Autodesk Fusion 360 part; units mm, degrees
sketch "Sketch7" plane through (0, 0, 0) normal (0, 1, 0) x (1, 0, 0)
  line L0 (2455.4576, -95.8693) -> (2455.4576, -76.2)
  line L1 (2455.4576, -76.2) -> (2651.76, 0)
  line L2 (2651.76, 0) -> (2706.624, 0)
  line L3 (2706.624, 0) -> (3456.432, -140.208)
  line L4 (3456.432, -140.208) -> (3535.68, -408.432)
  line L5 (3535.68, -408.432) -> (3066.288, -402.336)
  line L6 (3066.288, -402.336) -> (2455.4576, -95.8693)
extrude "Extrude5" add sketch "Sketch7" along normal blind 950.976
sketch "Sketch8" plane through (0, 0, 0) normal (1, 0, 0) x (0, 1, 0)
  line L0 (950.976, 426.72) -> (0, 426.72)
  line L1 (475.488, 426.72) -> (475.488, -243.84)
  line L2 (1005.84, 457.2) -> (-54.0718, 457.2)
  line L3 (-54.0718, 457.2) -> (-54.0718, -231.5284)
  line L4 (-54.0718, -231.5284) -> (1005.84, -231.5284)
  line L5 (1005.84, -231.5284) -> (1005.84, 457.2)
  line L6 (911.352, 27.432) -> (933.2048, 2.8476)
  line L7 (938.5836, 2.5312) -> (943.1535, 6.5933)
  line L8 (944.4292, 9.2894) -> (950.976, 173.736)
  line L9 (950.976, 173.736) -> (950.976, 391.668)
  line L10 (917.448, 391.668) -> (902.208, 176.784)
  line L11 (902.208, 176.784) -> (475.488, 176.784)
  arc A0 (950.976, 391.668) -> (917.448, 391.668) centre (934.212, 391.668) ccw
  line L12 (911.352, 27.432) -> (475.488, 27.432)
  arc A1 (933.2048, 2.8476) -> (938.5836, 2.5312) centre (936.0524, 5.3789) ccw
  arc A2 (943.1535, 6.5933) -> (944.4292, 9.2894) centre (940.6223, 9.4409) ccw
  line L13 (48.768, 176.784) -> (475.488, 176.784)
  line L14 (33.528, 391.668) -> (48.768, 176.784)
  arc A3 (33.528, 391.668) -> (0, 391.668) centre (16.764, 391.668) ccw
  line L15 (0, 173.736) -> (0, 391.668)
  line L16 (6.5468, 9.2894) -> (0, 173.736)
  arc A4 (6.5468, 9.2894) -> (7.8225, 6.5933) centre (10.3537, 9.4409) ccw
  line L17 (12.3924, 2.5312) -> (7.8225, 6.5933)
  arc A5 (12.3924, 2.5312) -> (17.7712, 2.8476) centre (14.9236, 5.3789) ccw
  line L18 (39.624, 27.432) -> (17.7712, 2.8476)
  line L19 (39.624, 27.432) -> (475.488, 27.432)
  dimension "d19" = 3.81
extrude "Extrude6" cut sketch "Sketch8" along normal blind 3962.4
ref_plane "WorkPlane3" through (3041.9851, 475.488, 481.584) normal (0, 0, 1) x (0, -1, 0)
sketch "Sketch10" plane through (0, 0, 481.584) normal (0, 0, 1) x (-1, 0, 0)
  line L0 (-2616.7317, -902.208) -> (-2616.7317, -48.768)
  line L1 (-2616.7317, -48.768) -> (-3467.2386, -48.768)
  line L2 (-3467.2386, -48.768) -> (-3467.2386, -902.208)
  line L3 (-3467.2386, -902.208) -> (-2616.7317, -902.208)
  line L4 (-2616.7317, -475.488) -> (-3627.1201, -475.488)
  line L5 (-2616.7317, -475.488) -> (-2616.7317, -932.688)
  line L6 (-2616.7317, -932.688) -> (-3467.2386, -902.208)
  line L7 (-3467.2386, -902.208) -> (-3467.2386, -475.488)
  line L8 (-2616.7317, -475.488) -> (-2616.7317, -18.288)
  line L9 (-2616.7317, -18.288) -> (-3467.2386, -48.768)
  line L10 (-3467.2386, -48.768) -> (-3467.2386, -475.488)
extrude "Extrude7" cut sketch "Sketch10" against normal blind 304.8 contours L3 L5 L6 | L1 L8 L9
Geometry: final body of the model. Coordinates: model frame, mm. A direction names the side the tool comes from. Give positions to 0.01 mm unless a question says otherwise; leave off trailing zeros. Loops run counter-clockwise (first coordinate to the right, second up) from the corner with the lowest first, then second, coordinate; pieces in that order, holes last. Notation, with made-up numbers: (-18, -3.75) -> (23, -3.75) arc R18 ccw to (23, 27.25) -> close; hole circle Ø11 at (48.25, 54.5). An arc over 180 degrees is marked (long way). Use CSV: the item, a comma, the result in double quotes.
(1) First-contact query: P1, Ø2, axis at y = 307.5, z = 103.5, coming from the -X side; P2, Ø8, axis at y = 648, z = 151.5, coming from the +X side; P3, Ø1.5, axis at x = 2607.5, z = 58, coming from the +Y side. Flat tips, straight axial feed; report the tip coordinate or a pass-through.
From the geometry:
P1,"x = 2468.67"
P2,"x = 3460.95"
P3,"y = 946.4"
(2) Ray query, line 1 along Z through (x, y) = (2748, 650.5); line 2 along Z through (x, y) = (2969, 797); line 3 along Y through (x, z) = (3460, 222.5). Return the intervals inside material, ascending. Write a range as [from, to].
From the geometry:
line 1,"[27.43, 176.78]"
line 2,"[49.06, 176.78]"
line 3,"[0, 45.53], [905.45, 950.98]"
(3) Cut plane C-C (y = 872). Output: boundary loops of the cut face in (x, z), plus the area to 3 significant figures.
From the geometry:
outline,"(2455.46, 76.2) -> (2581.09, 27.43) -> (2853.33, 27.43) -> (3456.43, 140.21) -> (3467.24, 176.78) -> (2616.73, 176.78) -> (2455.46, 95.87) -> close"
area,"106,000 mm^2"
(4) Cut plane D-D (z = 271). Output: boundary loops of the cut face in (x, y), plus the area to 3 significant figures.
From the geometry:
outline,"(2804.52, 0) -> (3495.08, 0) -> (3495.08, 42.09) -> (3280.79, 42.09) -> (2804.52, 25.02) -> close; (2804.52, 925.96) -> (3280.79, 908.89) -> (3495.08, 908.89) -> (3495.08, 950.98) -> (2804.52, 950.98) -> close"
area,"50,000 mm^2"
(5) Cut plane A-A (z = 197). Output: boundary loops of the cut face in (x, y).
From the geometry:
outline,"(2657.03, 0) -> (3473.21, 0) -> (3473.21, 47.33) -> (3427.23, 47.33) -> (2657.03, 19.73) -> close; (2657.03, 931.24) -> (3427.23, 903.64) -> (3473.21, 903.64) -> (3473.21, 950.98) -> (2657.03, 950.98) -> close"
(6) Cut plane B-B (x = 3328). Output: boundary loops of the cut face in (y, z).
From the geometry:
outline,"(0, 173.74) -> (2.29, 116.19) -> (948.69, 116.19) -> (950.98, 173.74) -> (950.98, 391.67) arc R16.76 ccw to (943.33, 405.73) -> (925.09, 405.73) arc R16.76 ccw to (917.45, 391.67) -> (907.2, 247.14) -> (907.2, 176.78) -> (43.78, 176.78) -> (43.78, 247.14) -> (33.53, 391.67) arc R16.76 ccw to (25.88, 405.73) -> (7.65, 405.73) arc R16.76 ccw to (0, 391.67) -> close"
(7) Pull-direction query (Y, two-part tool) for faces 1 (the face through (2841.502, 948.384, 108.633)), 2 (the face through (3048, 469, 176.784)), 3 (the face through (2528.88, 468.89, 47.7)); classes: released by +Y, released by -Y, zero draft, split by the parting line, or undercut.
From the geometry:
face 1,"released by +Y"
face 2,"undercut"
face 3,"zero draft"
(8) Access query for faces 4 (the face through (3337.84, 913.32, 333.48)), 5 (the face through (2715.303, 31.279, 18.043)), 6 (the face through (2841.5, 2.59, 108.63)). Directions: +Z, -Z, +X, -X, +Y, -Y. A direction counts if a zero-diameter tool reaches every point of the face in a straight line with its end or side. Return the directions, or none.
From the geometry:
face 4,"+Z, +X, -X"
face 5,"-Z, +X, -X"
face 6,"-Z, +X, -X, -Y"
